Source: CAD feature listing. Evaluate the final solid. Frame: model axes, mm. A direction names the side the tool comes from. Give positions to 0.01 mm unless a question says otherwise; leave off trailing zeros. Loops run counter-clockwise (first coordinate to the right, second up) from the corner with the lowest first, then second, coordinate; pieces in that order, holes last. Notation, with made-up numbers: (46, 46) -> (96, 46) arc R10 cw to (96, 59) -> close; hole circle Ø7 at (-7.5, -5). An arc over 180 degrees is marked (long way). Put each result on its own line as item: value.
```python
from build123d import *

# Parameters (mm, degrees)
SKETCH1_W                = 24
SKETCH1_H                = 52.5
SKETCH1_R                = 6.1
BOSS_EXTRUDE1_DEPTH      = 13.5
BOSS_EXTRUDE2_DEPTH      = 3
BOSS_EXTRUDE2_DEPTH_BACK = 2
SKETCH3_W                = 27
SKETCH3_H                = 18
BOSS_EXTRUDE3_DEPTH      = 15
SKETCH4_W                = 32
SKETCH4_H                = 12
CUT_EXTRUDE2_DEPTH       = 18
SKETCH6_W                = 65
SKETCH6_H                = 56
BOSS_EXTRUDE4_DEPTH      = 22
SKETCH7_R                = 3.1
CUT_EXTRUDE3_DEPTH       = 57
SKETCH8_W                = 17
SKETCH8_H                = 65
CUT_EXTRUDE4_DEPTH       = 17.5
SKETCH11_W               = 22.6
SKETCH11_H               = 12.25
CUT_EXTRUDE6_DEPTH       = 5
SKETCH12_W               = 17
SKETCH12_H               = 27
CUT_EXTRUDE7_DEPTH       = 39.5
SKETCH13_W               = 17
SKETCH13_H               = 65
CUT_EXTRUDE8_DEPTH       = 25.5
SKETCH16_W               = 15
SKETCH16_H               = 27
CUT_EXTRUDE9_DEPTH       = 6
SKETCH17_W               = 15
SKETCH17_H               = 12
BOSS_EXTRUDE5_DEPTH      = 5
BOSS_EXTRUDE5_DEPTH_BACK = 32
SKETCH19_W               = 21
SKETCH19_H               = 27
BOSS_EXTRUDE6_DEPTH      = 3.05
SKETCH20_W               = 1
SKETCH20_H               = 11.8
CUT_EXTRUDE11_DEPTH      = 47
SKETCH21_R               = 1.2
CUT_EXTRUDE12_DEPTH      = 10
SKETCH23_W               = 17
SKETCH23_H               = 13
BOSS_EXTRUDE7_DEPTH      = 4
SKETCH24_W               = 17
SKETCH24_H               = 13
BOSS_EXTRUDE8_DEPTH      = 4
SKETCH25_R               = 2.1
CUT_EXTRUDE14_DEPTH      = 74
SKETCH26_W               = 8
SKETCH26_H               = 4
CUT_EXTRUDE15_DEPTH      = 39.5
SKETCH27_W               = 3
SKETCH27_H               = 21.2
BOSS_EXTRUDE9_DEPTH      = 32.5
SKETCH28_R               = 1.3
CUT_EXTRUDE16_DEPTH      = 43


with BuildPart() as part:
    # Sketch1 → Boss-Extrude1 (new body, symmetric)
    with BuildSketch(Plane.XY):
        with Locations((12, 0)):
            Rectangle(SKETCH1_W, SKETCH1_H)
        with Locations((12, 14.25)):
            Circle(SKETCH1_R, mode=Mode.SUBTRACT)
        with Locations((12, -14.25)):
            Circle(SKETCH1_R, mode=Mode.SUBTRACT)
    extrude(amount=BOSS_EXTRUDE1_DEPTH, both=True)

    # Sketch2 → Boss-Extrude2 (add, two sides)
    with BuildSketch(Plane(origin=(0, 5.5, 0), x_dir=(1, 0, 0), z_dir=(0, 1, 0))) as boss_extrude2_sk:
        Polygon((-4, -7), (0, -7), (0, -15.75), (-15, -15.75), (-15, -7), (-11, -7), align=None)
        with BuildLine():
            Line((-11.25, -8.75), (-3.75, -8.75))
            ThreePointArc((-3.75, -8.75), (-2.25, -10.25), (-3.75, -11.75))
            Line((-3.75, -11.75), (-11.25, -11.75))
            ThreePointArc((-11.25, -11.75), (-12.75, -10.25), (-11.25, -8.75))
        make_face(mode=Mode.SUBTRACT)
        Polygon((-4, 7), (-11, 7), (-15, 7), (-15, 15.75), (0, 15.75), (0, 7), align=None)
        with BuildLine():
            ThreePointArc((-3.75, 8.75), (-2.25, 10.25), (-3.75, 11.75))
            Line((-3.75, 11.75), (-11.25, 11.75))
            ThreePointArc((-11.25, 11.75), (-12.75, 10.25), (-11.25, 8.75))
            Line((-11.25, 8.75), (-3.75, 8.75))
        make_face(mode=Mode.SUBTRACT)
    extrude(amount=BOSS_EXTRUDE2_DEPTH)
    extrude(boss_extrude2_sk.sketch, amount=-BOSS_EXTRUDE2_DEPTH_BACK)

    # Sketch3 → Boss-Extrude3 (add)
    with BuildSketch(Plane.ZY):
        Polygon((13.5, 26.25), (-13.5, 26.25), (-13.5, 12.5), (-8.75, 12.5), (8.75, 12.5), (13.5, 12.5), align=None)
        Polygon((8.75, 12.5), (-8.75, 12.5), (-8.75, 8.5), (-7, 8.5), (-7, 5.5), (7, 5.5), (7, 8.5), (8.75, 8.5), align=None)
        with Locations((0, -17.25)):
            Rectangle(SKETCH3_W, SKETCH3_H)
    extrude(amount=BOSS_EXTRUDE3_DEPTH)

    # Sketch4 → Cut-Extrude2 (cut)
    with BuildSketch(Plane.ZY.offset(15)):
        with Locations((0, 23.5)):
            Rectangle(SKETCH4_W, SKETCH4_H)
    extrude(amount=-CUT_EXTRUDE2_DEPTH, mode=Mode.SUBTRACT)

    # Sketch6 → Boss-Extrude4 (add)
    with BuildSketch(Plane.ZY.offset(15)):
        with Locations((0, 1.75)):
            Rectangle(SKETCH6_W, SKETCH6_H)
    extrude(amount=BOSS_EXTRUDE4_DEPTH)

    # Sketch7 → Cut-Extrude3 (cut, through all)
    with BuildSketch(Plane(origin=(0, 29.75, 0), x_dir=(1, 0, 0), z_dir=(0, 1, 0))):
        with Locations((-29, 23)):
            Circle(SKETCH7_R)
        with Locations((-29, -23)):
            Circle(SKETCH7_R)
    extrude(amount=-CUT_EXTRUDE3_DEPTH, mode=Mode.SUBTRACT)

    # Sketch8 → Cut-Extrude4 (cut)
    with BuildSketch(Plane(origin=(0, 29.75, 0), x_dir=(1, 0, 0), z_dir=(0, 1, 0))):
        with Locations((-28.5, 0)):
            Rectangle(SKETCH8_W, SKETCH8_H)
    extrude(amount=-CUT_EXTRUDE4_DEPTH, mode=Mode.SUBTRACT)

    # Sketch11 → Cut-Extrude6 (cut)
    with BuildSketch(Plane.ZY.offset(20)):
        with Locations((0, 23.625)):
            Rectangle(SKETCH11_W, SKETCH11_H)
    extrude(amount=-CUT_EXTRUDE6_DEPTH, mode=Mode.SUBTRACT)

    # Sketch12 → Cut-Extrude7 (cut, through all)
    with BuildSketch(Plane(origin=(0, 12.25, 0), x_dir=(1, 0, 0), z_dir=(0, 1, 0))):
        with Locations((-28.5, 0)):
            Rectangle(SKETCH12_W, SKETCH12_H)
    extrude(amount=-CUT_EXTRUDE7_DEPTH, mode=Mode.SUBTRACT)

    # Sketch13 → Cut-Extrude8 (cut)
    with BuildSketch(Plane.XZ.offset(26.25)):
        with Locations((-28.5, 0)):
            Rectangle(SKETCH13_W, SKETCH13_H)
    extrude(amount=-CUT_EXTRUDE8_DEPTH, mode=Mode.SUBTRACT)

    # Sketch16 → Cut-Extrude9 (cut)
    with BuildSketch(Plane(origin=(0, -8.25, 0), x_dir=(1, 0, 0), z_dir=(0, 1, 0))):
        with Locations((-7.5, 0)):
            Rectangle(SKETCH16_W, SKETCH16_H)
    extrude(amount=-CUT_EXTRUDE9_DEPTH, mode=Mode.SUBTRACT)

    # Sketch17 → Boss-Extrude5 (add, two sides)
    with BuildSketch(Plane(origin=(0, 0, -13.5), x_dir=(-1, 0, 0), z_dir=(0, 0, -1))) as boss_extrude5_sk:
        with Locations((7.5, -20.25)):
            Rectangle(SKETCH17_W, SKETCH17_H)
    extrude(amount=BOSS_EXTRUDE5_DEPTH)
    extrude(boss_extrude5_sk.sketch, amount=-BOSS_EXTRUDE5_DEPTH_BACK)

    # Sketch19 → Boss-Extrude6 (add)
    with BuildSketch(Plane(origin=(0, 26.25, 0), x_dir=(1, 0, 0), z_dir=(0, 1, 0))):
        with Locations((13.5, 0)):
            Rectangle(SKETCH19_W, SKETCH19_H)
    extrude(amount=BOSS_EXTRUDE6_DEPTH)

    # Sketch20 → Cut-Extrude11 (cut, through all)
    with BuildSketch(Plane.XY.offset(13.5)):
        with Locations((3.5, 23.4)):
            Rectangle(SKETCH20_W, SKETCH20_H)
    extrude(amount=-CUT_EXTRUDE11_DEPTH, mode=Mode.SUBTRACT)

    # Sketch21 → Cut-Extrude12 (cut)
    with BuildSketch(Plane(origin=(-15, 0, 0), x_dir=(0, 0, -1), z_dir=(1, 0, 0))):
        with Locations((-13.7, 23.4)):
            Circle(SKETCH21_R)
        with Locations((13.6, 23.4)):
            Circle(SKETCH21_R)
    extrude(amount=-CUT_EXTRUDE12_DEPTH, mode=Mode.SUBTRACT)

    # Sketch23 → Boss-Extrude7 (add)
    with BuildSketch(Plane(origin=(0, 0, -32.5), x_dir=(-1, 0, 0), z_dir=(0, 0, -1))):
        with Locations((28.5, 5.75)):
            Rectangle(SKETCH23_W, SKETCH23_H)
    extrude(amount=BOSS_EXTRUDE7_DEPTH)

    # Sketch24 → Boss-Extrude8 (add)
    with BuildSketch(Plane.XY.offset(32.5)):
        with Locations((-28.5, 5.75)):
            Rectangle(SKETCH24_W, SKETCH24_H)
    extrude(amount=BOSS_EXTRUDE8_DEPTH)

    # Sketch25 → Cut-Extrude14 (cut, through all)
    with BuildSketch(Plane(origin=(0, 0, -36.5), x_dir=(-1, 0, 0), z_dir=(0, 0, -1))):
        with Locations((28.902210775, 5.75)):
            Circle(SKETCH25_R)
    extrude(amount=-CUT_EXTRUDE14_DEPTH, mode=Mode.SUBTRACT)

    # Sketch26 → Cut-Extrude15 (cut, through all)
    with BuildSketch(Plane(origin=(0, 12.25, 0), x_dir=(1, 0, 0), z_dir=(0, 1, 0))):
        with Locations((-29, -30.5)):
            Rectangle(SKETCH26_W, SKETCH26_H)
        with Locations((-29, 30.5)):
            Rectangle(SKETCH26_W, SKETCH26_H)
    extrude(amount=-CUT_EXTRUDE15_DEPTH, mode=Mode.SUBTRACT)

    # Sketch27 → Boss-Extrude9 (add)
    with BuildSketch(Plane(origin=(0, 29.75, 0), x_dir=(1, 0, 0), z_dir=(0, 1, 0))):
        with Locations((-16.5, 21.9)):
            Rectangle(SKETCH27_W, SKETCH27_H)
    extrude(amount=BOSS_EXTRUDE9_DEPTH)

    # Sketch28 → Cut-Extrude16 (cut, through all)
    with BuildSketch(Plane.ZY.offset(18)):
        with Locations((-26.65, 54.95)):
            Circle(SKETCH28_R)
        with Locations((-17.05, 54.95)):
            Circle(SKETCH28_R)
    extrude(amount=-CUT_EXTRUDE16_DEPTH, mode=Mode.SUBTRACT)


solid = part.part
```
(1) Reachability of faces 1 (the flat face through (0, 10, 11)), 2 (the flat face through (-18, 24, 11.3)), 3 (the flat face through (-19, 29.75, -22)), 4 (the flat face through (-7, 6, 15.75)), 5 (the flat face through (-27, 7, 32.5)) from +Z, -Z, +X, -X, +Y, -Y: full face, straight path, thin tool, end or side. Return the list, or none.
Calculated:
face 1: +Z
face 2: -X, +Y
face 3: +Z, -Z, -X, +Y
face 4: +Z, +X, +Y
face 5: +Y, -Y
(2) Section B-B on y = 54.95. Return loops of the section in (x, z).
Calculated:
outline: (-18, -32.5) -> (-15, -32.5) -> (-15, -27.95) -> (-18, -27.95) -> close; (-18, -25.35) -> (-15, -25.35) -> (-15, -18.35) -> (-18, -18.35) -> close; (-18, -15.75) -> (-15, -15.75) -> (-15, -11.3) -> (-18, -11.3) -> close
(3) Section D-D on y = 15.5. Return loops of the section in (x, z), then the cut area to 3 significant figures.
Calculated:
outline: (-20, -32.5) -> (-15, -32.5) -> (-15, -13.5) -> (6.03, -13.5) -> (6.03, 13.5) -> (-15, 13.5) -> (-15, 32.5) -> (-20, 32.5) -> close; (17.97, -13.5) -> (24, -13.5) -> (24, 13.5) -> (17.97, 13.5) -> close
area: 1,060 mm²
(4) First-contact query: P1, Ø7, axis at x = -5.5, z = -6.5, coming from the +Y side; P2, Ø8.5, axis at x = -25, z = 19.5, coming from the -Y side; P3, Ø0.7, axis at y = 7, z = -14.5, coming from the +X side; P4, Ø8, axis at x = -6, z = -24.5, coming from the +Y side. Flat tips, straight axial feed; report the tip coordinate or a pass-through.
Calculated:
P1: stops at y = 17.5
P2: stops at y = -0.75
P3: stops at x = 0
P4: passes through
(5) Line query: probe 1 along Y at (x, z) = (-1.5, 9.5); probe 2 along Z at (x, y) = (-29, 8.5); probe 3 along Z at (x, y) = (-17, 23). Output: solid intervals per line, ascending. Write a range as from..to.
Calculated:
probe 1: y = -26.25..-14.25, 3.5..8.5, 12.5..17.5
probe 2: z = -36.5..-32.5, -28.5..-26.1, -19.9..-13.5, 13.5..19.9, 26.1..28.5, 32.5..36.5
probe 3: z = -32.5..-14.73, -12.47..-11.3, 11.3..12.57, 14.83..32.5
(6) Draft query along X for faces 6 (the flat face through (14, 29.3, 0)), 7 (the flat face through (0, 6, 15)), 8 (the cylindrical face through (-26.804, 5.842, 34.472)). Return one class per face: released by +X, released by -X, zero draft, split by the parting line, or undercut.
Calculated:
face 6: zero draft
face 7: released by +X
face 8: undercut
(7) Section C-C on z = 10.25. Return loops of the section in (x, y), then the cut area to 3 significant figures.
Calculated:
outline: (-20, -26.25) -> (24, -26.25) -> (24, 29.3) -> (4, 29.3) -> (4, 17.5) -> (-20, 17.5) -> close; hole (-15, -14.25) -> (0, -14.25) -> (0, 3.5) -> (-2.25, 3.5) -> (-2.25, 8.5) -> (0, 8.5) -> (0, 12.5) -> (-15, 12.5) -> (-15, 8.5) -> (-12.75, 8.5) -> (-12.75, 3.5) -> (-15, 3.5) -> close; hole circle Ø12.2 at (12, -14.25); hole circle Ø12.2 at (12, 14.25)
area: 1,550 mm²
(8) Section A-A on z = -23. Return loops of the section in (x, y).
Calculated:
outline: (-37, -0.75) -> (-32.1, -0.75) -> (-32.1, 12.25) -> (-37, 12.25) -> close; (-25.9, -0.75) -> (-20, -0.75) -> (-20, -26.25) -> (-15, -26.25) -> (-15, 62.25) -> (-18, 62.25) -> (-18, 29.75) -> (-20, 29.75) -> (-20, 12.25) -> (-25.9, 12.25) -> close
